For this review, take the finished solid that the model builds, in its own axes (mm). Face numbers are marked on the shaded views. A direction names the side the tool comes from. Round coordinates to 2 decimals unless told otherwise and drop trailing zeros. Loops run counter-clockwise (first coordinate to the right, second up) from the corner with the lowest first, then second, coordinate; pieces in that order, holes last.
1) Take a section at A-A (z = 0). State the section outline as (x, y) points, then the cut area to 3 significant figures.
2) Insertion check: pin 1 (4 mm diameter, centred on y = 12, z = 5.5, fed in from +X); pin 2 (12 mm diameter, centred on y = 27.5, z = -2.5, fed in from +X); pin 3 (2.5 mm diameter, centred on x = -15, z = 0, fed in from +Y); pin 4 (5 mm diameter, centred on x = -2, z = -4.5, fed in from -Y). Each pin has a flat end and moves straight along its axis. Give the tip position at first contact, or say it passes through.
3) Tool access review of the marked faces 1, 2 and 3: name each direction out of +Z, -Z, +X, -X, +Y, -Y from which nothing blocks a thin tool from reaching the whole face with its end or side.
4) Wall thickness on L1, parallel to Y at x = 13.5, z = -1.5; L2, parallel to X at y = 24, z = -5; L3, parallel to X at y = 32, z = 6: over which ranges is each line inside the solid? List them lowest first.
5) Take a section at D-D (y = 12.5). State the section outline as (x, z) points, then the cut area to 3 significant figures.
6) Mouldability with a two-part tool opening along X and no side actions: class the marked faces 4, 5, 6 and 7 as pulls with the +X half, pulls with the -X half, needs draft (parallel to the pull), parting line crosses it, or undercut.
7) Take a section at B-B (y = 26). State the section outline as (x, z) points.
8) Take a section at C-C (x = -6.5). State the section outline as (y, z) points.
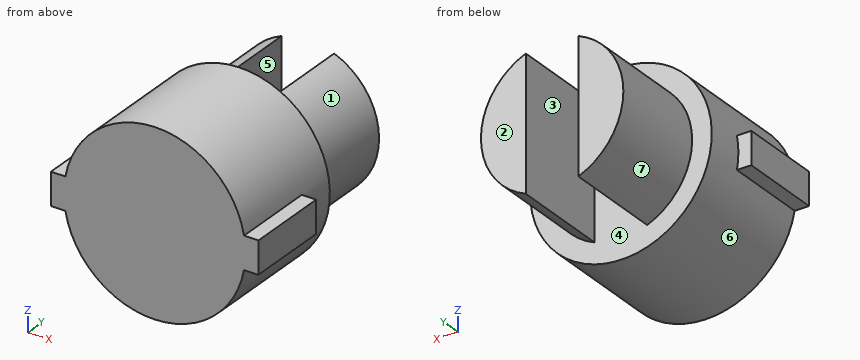
```python
from build123d import *

# Parameters (mm, degrees)
BOSS_EXTRUDE1_DEPTH   = 34.5
BOSS_EXTRUDE1_2_DEPTH = 34.5
SKETCH1_4_R           = 14
BOSS_EXTRUDE2_DEPTH   = 19
BOSS_EXTRUDE3_DEPTH   = 13


with BuildPart() as part:
    # Sketch1 → Boss-Extrude1 (new body)
    with BuildSketch(Plane(origin=(0, 0, 0), x_dir=(1, 0, 0), z_dir=(0, 1, 0))):
        with BuildLine():
            ThreePointArc((4.058218824, -10.202512434), (10.98, 0), (4.058218824, 10.202512434))
            Line((4.058218824, 10.202512434), (4.058218824, -10.202512434))
        make_face()
    extrude(amount=BOSS_EXTRUDE1_DEPTH)



with BuildPart() as body_2:
    # Sketch1 → Boss-Extrude1 2 (new body)
    with BuildSketch(Plane(origin=(0, 0, 0), x_dir=(1, 0, 0), z_dir=(0, 1, 0))):
        with BuildLine():
            Line((-4.043488658, -10.208359294), (-4.043488658, 10.208359294))
            ThreePointArc((-4.043488658, 10.208359294), (-10.98, 0), (-4.043488658, -10.208359294))
        make_face()
    extrude(amount=BOSS_EXTRUDE1_2_DEPTH)


with BuildPart() as part_1:
    add(part.part)

    add(body_2.part)  # Boss-Extrude2 merges body 2
    # Sketch1_4 → Boss-Extrude2 (add)
    with BuildSketch(Plane(origin=(0, 0, 0), x_dir=(1, 0, 0), z_dir=(0, 1, 0))):
        with Locations(Location((0, 0, 0), (0, 0, 270))):
            Circle(SKETCH1_4_R)
    extrude(amount=BOSS_EXTRUDE2_DEPTH)

    # Sketch1_5 → Boss-Extrude3 (add)
    with BuildSketch(Plane(origin=(0, 0, 0), x_dir=(1, 0, 0), z_dir=(0, 1, 0))):
        with BuildLine():
            Line((-16, -2.498244783), (-13.77529575, -2.498244783))
            ThreePointArc((-13.77529575, -2.498244783), (-13.999999886, 0.001783889), (-13.774658647, 2.501755217))
            Line((-13.774658647, 2.501755217), (-16, 2.501755217))
            Line((-16, 2.501755217), (-16, -2.498244783))
        make_face()
        with BuildLine():
            ThreePointArc((14, 0), (13.943710778, -1.254164961), (13.77529575, -2.498244783))
            Line((13.77529575, -2.498244783), (15.995322261, -2.498244783))
            Line((15.995322261, -2.498244783), (15.995322261, 2.5))
            Line((15.995322261, 2.5), (13.774977314, 2.5))
            ThreePointArc((13.774977314, 2.5), (13.943630847, 1.255053307), (14, 0))
        make_face()
    extrude(amount=BOSS_EXTRUDE3_DEPTH)


solid = part_1.part
```
Response:
1. outline: (-16, 0) - (16, 0) - (16, 13) - (14, 13) - (14, 19) - (10.98, 19) - (10.98, 34.5) - (4.06, 34.5) - (4.06, 19) - (-4.04, 19) - (-4.04, 34.5) - (-10.98, 34.5) - (-10.98, 19) - (-14, 19) - (-14, 13) - (-16, 13) - close
1. area: 799 mm2
2. pin 1: stops at x = 13.56
2. pin 2: stops at x = 10.98
2. pin 3: stops at y = 19
2. pin 4: stops at y = 0
3. face 1: +X, +Y
3. face 2: +Z, -Z, +X, -X, +Y
3. face 3: +Z, -Z, +Y
4. L1: y = 0 to 19
4. L2: x = -9.78 to -4.04, 4.06 to 9.78
4. L3: x = -9.2 to -4.04, 4.06 to 9.2
5. outline: (-16, -2.5) - (-13.77, -2.5) arc R14 ccw to (13.77, -2.5) - (16, -2.5) - (16, 2.5) - (13.78, 2.5) arc R14 ccw to (-13.78, 2.5) - (-16, 2.5) - close
5. area: 636 mm2
6. face 4: undercut
6. face 5: undercut
6. face 6: parting line crosses it
6. face 7: pulls with the -X half
7. outline: (-4.04, -10.21) - (-4.04, 10.21) arc R10.98 ccw to start; (4.06, -10.2) arc R10.98 ccw to (4.06, 10.2) - close
8. outline: (0, -12.4) - (19, -12.4) - (19, -8.85) - (34.5, -8.85) - (34.5, 8.85) - (19, 8.85) - (19, 12.4) - (0, 12.4) - close
